Read the model definition and answer for the solid it produces. Units are mm, in the model's axes. Give positions to 0.01 mm unless a question says otherwise; leave off trailing zeros. Order: outer loops, then holes, each group sorted by start corner. A loop starts at its lowest first (then second) coordinate and runs counter-clockwise, first axis right, second up. Notation, with made-up numbers: (48.5, 59.25) - (94.5, 59.25) arc R25 ccw to (94.5, 74.25) - close; hole circle Ø3 at (-31, 73). An arc over 180 degrees is marked (long way). Write item = value, one per line.
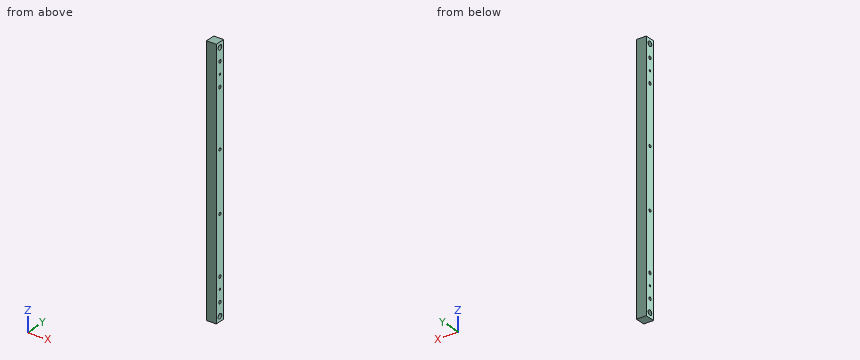
```python
from build123d import *

# Parameters (mm, degrees)
SKETCH1_W               = 25.4
SKETCH1_H               = 25.4
BOSS_EXTRUDE1_DEPTH     = 660.4
SKETCH2_R               = 6.35
CUT_EXTRUDE4_DEPTH      = 26.4
CUT_EXTRUDE4_DEPTH_BACK = 1
SKETCH3_R               = 3.97
SKETCH3_R_2             = 2.55
CUT_EXTRUDE5_DEPTH      = 26.4
SKETCH10_R              = 3.5
CUT_EXTRUDE6_DEPTH      = 26.4


with BuildPart() as part:
    # Sketch1 → Boss-Extrude1 (new body)
    with BuildSketch(Plane.XY):
        Rectangle(SKETCH1_W, SKETCH1_H)
    extrude(amount=BOSS_EXTRUDE1_DEPTH)

    # Sketch2 → Cut-Extrude4 (cut, two sides)
    with BuildSketch(Plane(origin=(-12.7, 0, 0), x_dir=(0, 0, -1), z_dir=(1, 0, 0))) as cut_extrude4_sk:
        with Locations((-12.7, 0)):
            Circle(SKETCH2_R)
        with Locations((-647.7, 0)):
            Circle(SKETCH2_R)
    extrude(amount=CUT_EXTRUDE4_DEPTH, mode=Mode.SUBTRACT)
    extrude(cut_extrude4_sk.sketch, amount=-CUT_EXTRUDE4_DEPTH_BACK, mode=Mode.SUBTRACT)

    # Sketch3 → Cut-Extrude5 (cut, through all)
    with BuildSketch(Plane.ZY.offset(12.7)):
        with Locations((554.0375, 0)):
            Circle(SKETCH3_R)
        with Locations((106.3625, 0)):
            Circle(SKETCH3_R)
        with Locations((614.3625, 0)):
            Circle(SKETCH3_R)
        with Locations((584.2, 0)):
            Circle(SKETCH3_R_2)
        with Locations((46.0375, 0)):
            Circle(SKETCH3_R)
        with Locations((76.2, 0)):
            Circle(SKETCH3_R_2)
    extrude(amount=-CUT_EXTRUDE5_DEPTH, mode=Mode.SUBTRACT)

    # Sketch10 → Cut-Extrude6 (cut, through all)
    with BuildSketch(Plane.ZY.offset(12.7)):
        with Locations((406.4, 0)):
            Circle(SKETCH10_R)
        with Locations((254, 0)):
            Circle(SKETCH10_R)
    extrude(amount=-CUT_EXTRUDE6_DEPTH, mode=Mode.SUBTRACT)


solid = part.part
```
1. Section B-B (x = 1.25) is taken. Count the separate pieces of the cut face and the enclosed holes in it, and give its area (3 significant figures).
Recorded:
separate_pieces = 1
enclosed_holes = 10
area = 16,200 mm^2
2. Section A-A (z = 647.7) is taken. Determine the outline of the cut face in (x, y).
Recorded:
outline = (-12.7, -12.7) - (12.7, -12.7) - (12.7, -6.35) - (-12.7, -6.35) - close; (-12.7, 6.35) - (12.7, 6.35) - (12.7, 12.7) - (-12.7, 12.7) - close
3. Straight lines are drawn through the part: L1, parallel to Y at x = -2.5, z = 76.2; L2, parallel to Y at x = -3, z = 647.7. For each, find the intervals that lie inside material, in ascending order. Write a range as [from, to].
Recorded:
L1 = [-12.7, -2.55], [2.55, 12.7]
L2 = [-12.7, -6.35], [6.35, 12.7]
